Design review of the part built by this model. Coordinates are the model's own, in mm. Round coordinates to 2 decimals unless told otherwise and drop trailing zeros. Loops run counter-clockwise (first coordinate to the right, second up) from the corner with the lowest first, then second, coordinate; pieces in that order, holes last. Notation, with made-up numbers: (71.5, 20.5) - (103.5, 20.5) arc R34 cw to (103.5, 57.5) - close; hole circle Ø10 at (-36.5, 33). An arc over 180 degrees is marked (long way). Use one line per item in the form item = value. Start each with the question number.
(1) We need section A-A, the plane y = 1.05. Give the number of separate pieces and of enclosed holes in the cut face, then the cut area to 3 significant figures.
(2) We need section C-C, the plane z = -217. Write out the cut boundary in (x, y) (3 decimals).
(3) For pin 1 (3 mm diameter, centred on x = 101.6, z = -9.525, fed in from -Y), flat-tipped, find the tip position at first contact; note if it passes through.
(4) We need section B-B, the plane z = -122.5. Write out the cut boundary in (x, y) (3 decimals), then the cut area to 3 significant figures.
(5) Wall thickness on probe 1 along Z at (x, y) = (111, 1.65); probe 2 along X at (y, z) = (2.2, -130.5); probe 3 along X at (y, z) = (0.55, -249.5): over which ranges is each line inside the solid? List them lowest first. Write a range as [from, to].
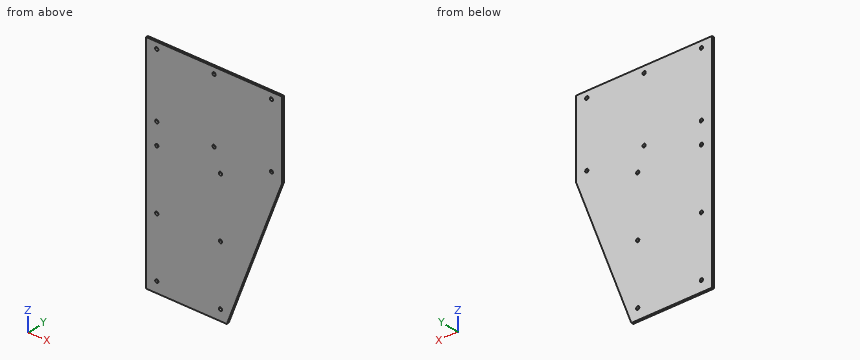
from build123d import *

# Parameters (mm, degrees)
SKETCH1_R           = 2.4257
BOSS_EXTRUDE1_DEPTH = 3.175


with BuildPart() as part:
    # Sketch1 → Boss-Extrude1 (new body)
    with BuildSketch(Plane(origin=(0, 0, 0), x_dir=(1, 0, 0), z_dir=(0, 1, 0))):
        Polygon((0, 0), (203.2, 0), (203.2, 114.3), (120.65, 330.2), (0, 330.2), align=None)
        with Locations(Location((15.875, 9.525, 0), (0, 0, 270))):
            Circle(SKETCH1_R, mode=Mode.SUBTRACT)
        with Locations(Location((101.6, 9.525, 0), (0, 0, 270))):
            Circle(SKETCH1_R, mode=Mode.SUBTRACT)
        with Locations(Location((187.325, 9.525, 0), (0, 0, 270))):
            Circle(SKETCH1_R, mode=Mode.SUBTRACT)
        with Locations(Location((15.875, 104.775, 0), (0, 0, 270))):
            Circle(SKETCH1_R, mode=Mode.SUBTRACT)
        with Locations(Location((187.325, 104.775, 0), (0, 0, 270))):
            Circle(SKETCH1_R, mode=Mode.SUBTRACT)
        with Locations(Location((101.6, 104.775, 0), (0, 0, 270))):
            Circle(SKETCH1_R, mode=Mode.SUBTRACT)
        with Locations(Location((15.875, 136.525, 0), (0, 0, 270))):
            Circle(SKETCH1_R, mode=Mode.SUBTRACT)
        with Locations(Location((111.125, 136.525, 0), (0, 0, 270))):
            Circle(SKETCH1_R, mode=Mode.SUBTRACT)
        with Locations(Location((15.875, 225.425, 0), (0, 0, 270))):
            Circle(SKETCH1_R, mode=Mode.SUBTRACT)
        with Locations(Location((15.875, 314.325, 0), (0, 0, 270))):
            Circle(SKETCH1_R, mode=Mode.SUBTRACT)
        with Locations(Location((111.125, 225.425, 0), (0, 0, 270))):
            Circle(SKETCH1_R, mode=Mode.SUBTRACT)
        with Locations(Location((111.125, 314.325, 0), (0, 0, 270))):
            Circle(SKETCH1_R, mode=Mode.SUBTRACT)
    extrude(amount=BOSS_EXTRUDE1_DEPTH)


solid = part.part
Data:
q1.separate_pieces = 1
q1.enclosed_holes = 12
q1.area = 58,000 mm^2
q2.outline = (0, 0) - (163.932, 0) - (163.932, 3.175) - (0, 3.175) - close
q3.pin_1 = through
q4.outline = (0, 0) - (200.065, 0) - (200.065, 3.175) - (0, 3.175) - close
q4.area = 635 mm^2
q5.probe_1 = [-330.2, -316.75], [-311.9, -227.85], [-223, -138.95], [-134.1, 0]
q5.probe_2 = [0, 197.01]
q5.probe_3 = [0, 151.51]
